from build123d import *

# Parameters (mm, degrees)
SKETCH1_W           = 250
SKETCH1_H           = 250
BOSS_EXTRUDE1_DEPTH = 60
SKETCH2_W           = 250
SKETCH2_H           = 50.233662696
BOSS_EXTRUDE2_DEPTH = 1370
SKETCH3_W           = 250
SKETCH3_H           = 152.663953539
BOSS_EXTRUDE3_DEPTH = 700


with BuildPart() as part:
    # Sketch1 → Boss-Extrude1 (new body)
    with BuildSketch(Plane.XY):
        with Locations((-125, 125)):
            Rectangle(SKETCH1_W, SKETCH1_H)
    extrude(amount=BOSS_EXTRUDE1_DEPTH)

    # Sketch2 → Boss-Extrude2 (add)
    with BuildSketch(Plane.XY.offset(60)):
        with Locations((-125, 25.116831348)):
            Rectangle(SKETCH2_W, SKETCH2_H)
    extrude(amount=BOSS_EXTRUDE2_DEPTH)

    # Sketch3 → Boss-Extrude3 (add)
    with BuildSketch(Plane(origin=(0, 50.233662696, 0), x_dir=(1, 0, 0), z_dir=(0, 1, 0))):
        with Locations((-125, -1353.668023231)):
            Rectangle(SKETCH3_W, SKETCH3_H)
    extrude(amount=BOSS_EXTRUDE3_DEPTH)


solid = part.part
The model under review builds one solid part; all positions refer to its coordinate system, in mm. A direction names the side the tool comes from. Round coordinates to 2 decimals unless told otherwise and drop trailing zeros. Loops run counter-clockwise (first coordinate to the right, second up) from the corner with the lowest first, then second, coordinate; pieces in that order, holes last. Notation, with made-up numbers: (-10.75, -31.75) -> (48.25, -31.75) arc R18 ccw to (48.25, -25.75) -> close; hole circle Ø1 at (13, -26.75). An arc over 180 degrees is marked (long way). Answer as CSV lines item,"result".
1) Tool access review of faces 1 (the face through (-250, 40, 1036)), 2 (the face through (-127, 50.234, 660)), 3 (the face through (-127, 250, 30)): name each direction out of +Z, -Z, +X, -X, +Y, -Y from which nothing blocks a thin tool from reaching the whole face with its end or side.
Geometry results:
face 1,"+Z, -Z, -X, +Y, -Y"
face 2,"+X, -X, +Y"
face 3,"-Z, +X, -X, +Y"
2) Add section C-C on z = 1181. Write out the cut boundary in (x, y), plus the area to 3 significant figures.
Geometry results:
outline,"(-250, 0) -> (0, 0) -> (0, 50.23) -> (-250, 50.23) -> close"
area,"12,600 mm²"
3) For P1, Ø10, axis at x = -180.5, z = 1072.5, coming from the -Y side; P2, Ø5, axis at x = -124, y = 261, coming from the -Z side; P3, Ø5, axis at x = -215, z = 343.5, coming from the +Y side, all flat-tipped, find the tip position at first contact; note any pin that passes through.
Geometry results:
P1,"stops at y = 0"
P2,"stops at z = 1277.34"
P3,"stops at y = 50.23"
4) Add section A-A on y = 231.5. Write out the cut boundary in (x, z).
Geometry results:
outline,"(-250, 0) -> (0, 0) -> (0, 60) -> (-250, 60) -> close; (-250, 1277.34) -> (0, 1277.34) -> (0, 1430) -> (-250, 1430) -> close"
5) To check wall thickness, follow line 1 along Z through (x, y) = (-28.5, 111); line 2 along Y through (x, z) = (-137, 805); line 3 along Z through (x, y) = (-18, 565). State the ranges of each line that lie inside material, in increasing order. Write a range as from..to.
Geometry results:
line 1,"z = 0..60, 1277.34..1430"
line 2,"y = 0..50.23"
line 3,"z = 1277.34..1430"
6) Add section B-B on x = -142.5. Write out the cut boundary in (y, z), plus the area to 3 significant figures.
Geometry results:
outline,"(0, 0) -> (250, 0) -> (250, 60) -> (50.23, 60) -> (50.23, 1277.34) -> (750.23, 1277.34) -> (750.23, 1430) -> (0, 1430) -> close"
area,"191,000 mm²"
